Check sheet for the modelled part. Datum: model origin and axes. Units: mm. A direction names the side the tool comes from. Coordinates: 2 decimals unless noted, no trailing zeros. Loops run counter-clockwise (first coordinate to the right, second up) from the corner with the lowest first, then second, coordinate; pieces in that order, holes last.
```python
from build123d import *

# Parameters (mm, degrees)
F1_DEPTH = 25.4


with BuildPart() as f1:
    # F0 (on Front) → F1 (new body)
    with BuildSketch(Plane.XZ):
        with BuildLine():
            ThreePointArc((19.284791, 16.530482), (16.762226, 16.687837), (16.616092, 19.211078))
            ThreePointArc((16.616092, 19.211078), (11.870376, 22.455605), (6.516592, 24.549828))
            Line((6.516592, 24.549828), (7.06953, 27.028912))
            Line((7.06953, 27.028912), (5.086263, 27.471263))
            Line((5.086263, 27.471263), (4.533324, 24.992178))
            ThreePointArc((4.533324, 24.992178), (2.781418, 25.247252), (1.016, 25.379672))
            Line((1.016, 25.379672), (1.016, 27.919672))
            Line((1.016, 27.919672), (-1.016, 27.919672))
            Line((-1.016, 27.919672), (-1.016, 25.379672))
            ThreePointArc((-1.016, 25.379672), (-2.781418, 25.247252), (-4.533324, 24.992178))
            Line((-4.533324, 24.992178), (-5.086263, 27.471263))
            Line((-5.086263, 27.471263), (-7.06953, 27.028912))
            Line((-7.06953, 27.028912), (-6.516592, 24.549828))
            ThreePointArc((-6.516592, 24.549828), (-11.870376, 22.455605), (-16.616092, 19.211078))
            ThreePointArc((-16.616092, 19.211078), (-16.762226, 16.687837), (-19.284791, 16.530482))
            ThreePointArc((-19.284791, 16.530482), (-21.815816, 13.00885), (-23.710856, 9.107979))
            Line((-23.710856, 9.107979), (-26.248305, 10.082682))
            Line((-26.248305, 10.082682), (-27.040335, 8.020787))
            Line((-27.040335, 8.020787), (-24.413065, 7.011581))
            ThreePointArc((-24.413065, 7.011581), (-24.787675, 5.543569), (-25.074094, 4.055834))
            Line((-25.074094, 4.055834), (-27.880973, 4.261933))
            Line((-27.880973, 4.261933), (-28.042721, 2.059081))
            Line((-28.042721, 2.059081), (-25.331804, 1.860028))
            ThreePointArc((-25.331804, 1.860028), (-25.4, 0), (-25.331804, -1.860028))
            Line((-25.331804, -1.860028), (-28.042721, -2.059081))
            Line((-28.042721, -2.059081), (-27.880973, -4.261933))
            Line((-27.880973, -4.261933), (-25.074094, -4.055834))
            ThreePointArc((-25.074094, -4.055834), (-24.787675, -5.543569), (-24.413065, -7.011581))
            Line((-24.413065, -7.011581), (-27.040335, -8.020787))
            Line((-27.040335, -8.020787), (-26.248305, -10.082682))
            Line((-26.248305, -10.082682), (-23.710856, -9.107979))
            ThreePointArc((-23.710856, -9.107979), (-21.815816, -13.00885), (-19.284791, -16.530482))
            ThreePointArc((-19.284791, -16.530482), (-16.762226, -16.687837), (-16.616092, -19.211078))
            ThreePointArc((-16.616092, -19.211078), (-9.339997, -23.620424), (-1.016, -25.379672))
            Line((-1.016, -25.379672), (-1.016, -27.919672))
            Line((-1.016, -27.919672), (1.016, -27.919672))
            Line((1.016, -27.919672), (1.016, -25.379672))
            ThreePointArc((1.016, -25.379672), (9.339997, -23.620424), (16.616092, -19.211078))
            ThreePointArc((16.616092, -19.211078), (16.762226, -16.687837), (19.284791, -16.530482))
            ThreePointArc((19.284791, -16.530482), (23.039789, -10.692432), (25.074094, -4.055834))
            Line((25.074094, -4.055834), (27.880973, -4.261933))
            Line((27.880973, -4.261933), (28.042721, -2.059081))
            Line((28.042721, -2.059081), (25.331804, -1.860028))
            ThreePointArc((25.331804, -1.860028), (25.4, 0), (25.331804, 1.860028))
            Line((25.331804, 1.860028), (28.042721, 2.059081))
            Line((28.042721, 2.059081), (27.880973, 4.261933))
            Line((27.880973, 4.261933), (25.074094, 4.055834))
            ThreePointArc((25.074094, 4.055834), (23.039789, 10.692432), (19.284791, 16.530482))
        make_face()
        with BuildLine():
            ThreePointArc((-11.896721, 4.445), (-8.980256, 8.980256), (-4.445, 11.896721))
            ThreePointArc((-4.445, 11.896721), (0, 12.7), (4.445, 11.896721))
            ThreePointArc((4.445, 11.896721), (8.980256, -8.980256), (-11.896721, -4.445))
            Line((-11.896721, -4.445), (-19.516721, -4.445))
            Line((-19.516721, -4.445), (-19.516721, 4.445))
            Line((-19.516721, 4.445), (-11.896721, 4.445))
        make_face(mode=Mode.SUBTRACT)
    extrude(amount=F1_DEPTH)


solid = f1.part
```
1) Section check D-D on z = 23. Enter the section's corners in (x, y).
Answer sheet:
outline: (-10.78, -25.4) - (10.78, -25.4) - (10.78, 0) - (-10.78, 0) - close
2) Section check C-C on x = -20.5. Enter the section's corners in (y, z), plus the area to 3 significant figures.
Answer sheet:
outline: (-25.4, -15) - (0, -15) - (0, 15) - (-25.4, 15) - close
area: 762 mm2
3) Mould release check, pull along X, two halves, no side actions. Record for faces 6 (the flat face through (-26.65, -12.52, -9.04)), 7 (the flat face through (-1.016, -13, 27)), 8 (the flat face through (6.79, -12.52, 25.77)), 9 (the flat face through (0, -13, 27.92)): +X half, -X half, draft (parallel to the pull), parting line (faces both ways), or undercut.
Answer sheet:
face 6: -X half
face 7: undercut
face 8: +X half
face 9: draft
4) Section check A-A on x = 0. Enter the section's corners in (y, z).
Answer sheet:
outline: (-25.4, -27.92) - (0, -27.92) - (0, -12.7) - (-25.4, -12.7) - close; (-25.4, 12.7) - (0, 12.7) - (0, 27.92) - (-25.4, 27.92) - close
5) Scan lines: line 1 (X direction, y = -15.25, z = 0); line 2 (Z direction, x = 0, y = -15.5); line 3 (Z direction, x = -18.5, y = -6.5) (3 decimals). Record each from-to range of solid material in increasing order.
Answer sheet:
line 1: x = -25.4 to -19.52, 12.7 to 25.4
line 2: z = -27.92 to -12.7, 12.7 to 27.92
line 3: z = -16.167 to -4.445, 4.445 to 16.167
6) Set-up check for faces 1 (the flat face through (1.016, -13, -27)), 2 (the flat face through (-16, -13, 4.445)), 3 (the flat face through (-25.745, -12.522, 7.523)), 4 (the flat face through (4.814, -12.522, 26.249)), 5 (the flat face through (26.458, -12.522, -4.157)): record each of +Z, -Z, +X, -X, +Y, -Y from which the full face is reachable in a straight line by a thin tool's end or side.
Answer sheet:
face 1: -Z, +X, +Y, -Y
face 2: +Y, -Y
face 3: -X, +Y, -Y
face 4: +Z, +Y, -Y
face 5: -Z, +Y, -Y
7) Section check B-B on z = 0. Enter the section's corners in (x, y), plus the area to 3 significant figures.
Answer sheet:
outline: (-25.4, -25.4) - (-19.52, -25.4) - (-19.52, 0) - (-25.4, 0) - close; (12.7, -25.4) - (25.4, -25.4) - (25.4, 0) - (12.7, 0) - close
area: 472 mm2
8) Depth check by flat-ended pin: pin 1 (10 mm diameter, centred on x = 21.5, y = -12, fed in from +Z); pin 2 (2 mm diameter, centred on x = 14.5, y = -14, fed in from -Z); pin 3 (1.3 mm diameter, centred on y = -17.5, z = 26.5, fed in from -X). Enter the tip coordinate at first touch or a pass-through.
Answer sheet:
pin 1: stops at z = 19.31
pin 2: stops at z = -21.52
pin 3: stops at x = -7.07
